Geometry: final body of the model. Coordinates: model frame, mm. Face numbers are marked on the shaded views. A direction names the side the tool comes from. Round coordinates to 2 decimals unless told otherwise and drop trailing zeros. Order: outer loops, then holes, each group sorted by start corner. A loop starts at its lowest first (then second) coordinate and runs counter-clockwise, first axis right, second up. Notation, with made-up numbers: (53.5, -7) -> (82.5, -7) arc R33 ccw to (82.5, 26) -> close; hole circle Ø3 at (53.5, 57.25). An arc over 180 degrees is marked (long way). Put each result on its own line as item: value.
```python
from build123d import *

# Parameters (mm, degrees)
CUT_EXTRUDE1_DEPTH = 1
SKETCH4_R          = 1.443375673
CUT_EXTRUDE2_DEPTH = 0.5
CUT_EXTRUDE2_DRAFT = -45


with BuildPart() as part:
    # Sketch2 → Revolve1 (revolve)
    with BuildSketch(Plane(origin=(0, 0, 0), x_dir=(0, 0, -1), z_dir=(1, 0, 0)), mode=Mode.PRIVATE) as revolve1_sk:
        Polygon((-7.35, 2.75), (-4.65, 2.75), (-4.5, 2.6), (-4.5, 1.5), (7, 1.5), (7.5, 1), (7.5, 0), (-7.5, 0), (-7.5, 2.6), align=None)
    revolve(revolve1_sk.sketch.rotate(Axis((0, 0, -7.5), (0, 0, 1)), 90), axis=Axis((0, 0, -7.5), (0, 0, 1)))

    # Sketch3 → Cut-Extrude1 (cut)
    with BuildSketch(Plane.XY.offset(7.5)):
        Polygon((0.721687836, 1.25), (-0.721687836, 1.25), (-1.443375673, 0), (-0.721687836, -1.25), (0.721687836, -1.25), (1.443375673, 0), align=None)
    extrude(amount=-CUT_EXTRUDE1_DEPTH, mode=Mode.SUBTRACT)


with BuildPart() as cut_extrude2_tool:
    # Sketch4 → Cut-Extrude2 (with draft: the straight prism first)
    with BuildSketch(Plane.XY.offset(7.5)):
        Circle(SKETCH4_R)
    extrude(amount=-CUT_EXTRUDE2_DEPTH)
    # Cut-Extrude2: the draft: its side faces are tilted about the plane it starts from
    cut_extrude2_sides = [cut_extrude2_tool.faces().sort_by_distance(p)[0] for p in [
        (-1.443375673, 0, 7.25),
    ]]
    draft(cut_extrude2_sides, Plane.XY.offset(7.5), CUT_EXTRUDE2_DRAFT)


with BuildPart() as part_1:
    add(part.part)

    # Cut-Extrude2: cut by cut_extrude2_tool
    add(cut_extrude2_tool.part, mode=Mode.SUBTRACT)


solid = part_1.part
```
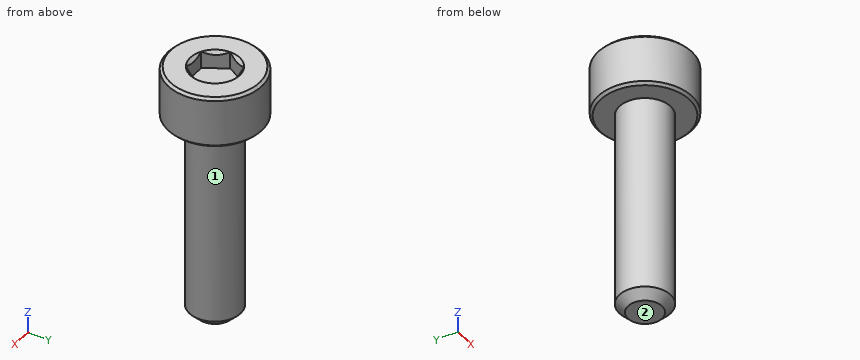
1. Cut plane A-A on x = 0. Return loops of the section in (y, z), and give its area (3 significant figures).
Ans:
outline: (-2.75, 4.65) -> (-2.6, 4.5) -> (-1.5, 4.5) -> (-1.5, -7) -> (-1, -7.5) -> (1, -7.5) -> (1.5, -7) -> (1.5, 4.5) -> (2.6, 4.5) -> (2.75, 4.65) -> (2.75, 7.35) -> (2.6, 7.5) -> (1.44, 7.5) -> (1.25, 7.31) -> (1.25, 6.5) -> (-1.25, 6.5) -> (-1.25, 7.31) -> (-1.44, 7.5) -> (-2.6, 7.5) -> (-2.75, 7.35) -> close
area: 49.7 mm²
2. Set-up query: the marked faces 1 and 2. Return all of +Z, -Z, +X, -X, +Y, -Y with unobstructed straight access to the full face (end or side cutting, diameter ignored); none if empty.
Ans:
face 1: -Z
face 2: -Z, +X, -X, +Y, -Y
3. Contact query for flat-ended pins moving along their axis: P1, Ø3, axis at y = -2, z = 1.5, coming from the +X side; P2, Ø1.5, axis at y = -1, z = 1, coming from the -X side; P3, Ø3, axis at y = -1, z = -0.5, coming from the +X side. Output: stop coordinate, or through.
Ans:
P1: x = 1.41
P2: x = -1.48
P3: x = 1.5
4. Material intervals for probe 1 along X at (y, z) = (-0.1, -4.75); probe 2 along Z at (x, y) = (-0.8, 1.45); probe 3 along Y at (x, z) = (-1.5, 6.5), sorted ascending.
Ans:
probe 1: -1.5 to 1.5
probe 2: 4.5 to 7.5
probe 3: -2.3 to 2.3
5. Cut plane B-B on z = -2.25. Return loops of the section in (x, y).
Ans:
outline: circle Ø3 at (0, 0)
